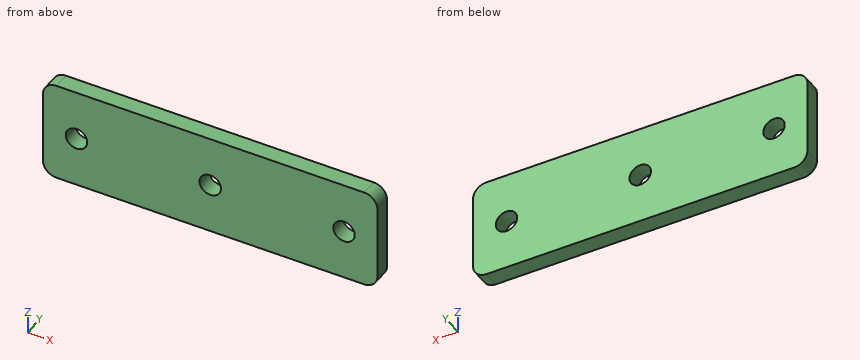
```python
from build123d import *

# Parameters (mm, degrees)
SKETCH_1_W          = 50
SKETCH_1_H          = 15
EXTRUDE_1_DEPTH     = 2.5
SKETCH_2_R          = 1.6
CUT_EXTRUDE_1_DEPTH = 27.220221204
FILLET_1_R          = 2


with BuildPart() as part:
    # 草图1 → 凸台-拉伸1 (new body)
    with BuildSketch(Plane(origin=(0, 0, 0), x_dir=(1, 0, 0), z_dir=(0, 1, 0))):
        Rectangle(SKETCH_1_W, SKETCH_1_H)
    extrude(amount=EXTRUDE_1_DEPTH)

    # 草图2 → 切除-拉伸1 (cut, through all)
    with BuildSketch(Plane(origin=(0, 2.5, 0), x_dir=(1, 0, 0), z_dir=(0, 1, 0))):
        with Locations(Location((0, 0, 0), (0, 0, 270))):
            Circle(SKETCH_2_R)
        with Locations(Location((-20, 0, 0), (0, 0, 270))):
            Circle(SKETCH_2_R)
        with Locations(Location((20, 0, 0), (0, 0, 270))):
            Circle(SKETCH_2_R)
    extrude(amount=-CUT_EXTRUDE_1_DEPTH, mode=Mode.SUBTRACT)

    # 圆角1
    fillet_1_edges = [part.edges().sort_by_distance(p)[0] for p in [
        (25, 1.25, 7.5),
        (-25, 1.25, 7.5),
        (-25, 1.25, -7.5),
        (25, 1.25, -7.5),
    ]]
    fillet(fillet_1_edges, radius=FILLET_1_R)


solid = part.part
```
The listing builds one solid part. Answer for the finished solid, in the listing's coordinates (mm). Give positions to 0.01 mm unless a question says otherwise; leave off trailing zeros. Write each loop counter-clockwise with the first axis right and the second up, starting at its lowest first coordinate (ties: lowest second). Pieces come first, ordered by that corner, then holes. Notation, with made-up numbers: (40.25, -34) -> (75.25, -34) arc R14 cw to (75.25, -8) -> close; hole circle Ø3 at (88, -21). An arc over 180 degrees is marked (long way). Write item = value, one per line. Start each with the question number.
1) The part is cut by section D-D, the plane x = 21. Determine the outline of the cut face in (y, z).
2) The part is cut by section C-C, the plane y = 1.75. Determine the outline of the cut face in (x, z), and give its area (3 significant figures).
3) The part is cut by section A-A, the plane x = -20. Determine the outline of the cut face in (y, z).
4) The part is cut by section B-B, the plane z = 0. Determine the outline of the cut face in (x, y).
5) Straight lines are drawn through the part: line 1 along X through (y, z) = (1.45, 0); line 2 along X through (y, z) = (1.2, -1.25). For each, find the intervals that lie inside material, in ascending order.
Solutions:
q1.outline = (0, -7.5) -> (2.5, -7.5) -> (2.5, -1.25) -> (0, -1.25) -> close; (0, 1.25) -> (2.5, 1.25) -> (2.5, 7.5) -> (0, 7.5) -> close
q2.outline = (-25, -5.5) arc R2 ccw to (-23, -7.5) -> (23, -7.5) arc R2 ccw to (25, -5.5) -> (25, 5.5) arc R2 ccw to (23, 7.5) -> (-23, 7.5) arc R2 ccw to (-25, 5.5) -> close; hole circle Ø3.2 at (-20, 0); hole circle Ø3.2 at (0, 0); hole circle Ø3.2 at (20, 0)
q2.area = 722 mm²
q3.outline = (0, -7.5) -> (2.5, -7.5) -> (2.5, -1.6) -> (0, -1.6) -> close; (0, 1.6) -> (2.5, 1.6) -> (2.5, 7.5) -> (0, 7.5) -> close
q4.outline = (-25, 0) -> (-21.6, 0) -> (-21.6, 2.5) -> (-25, 2.5) -> close; (-18.4, 0) -> (-1.6, 0) -> (-1.6, 2.5) -> (-18.4, 2.5) -> close; (1.6, 0) -> (18.4, 0) -> (18.4, 2.5) -> (1.6, 2.5) -> close; (21.6, 0) -> (25, 0) -> (25, 2.5) -> (21.6, 2.5) -> close
q5.line_1 = -25 to -21.6, -18.4 to -1.6, 1.6 to 18.4, 21.6 to 25
q5.line_2 = -25 to -21, -19 to -1, 1 to 19, 21 to 25
